```python
from build123d import *

# Parameters (mm, degrees)
SKETCH_1_W           = 88
SKETCH_1_H           = 58
EXTRUDE_1_DEPTH      = 18.8
SKETCH_2_W           = 7
SKETCH_2_H           = 7
CUT_EXTRUDE_1_DEPTH  = 15
SKETCH_3_R           = 1.55
CUT_EXTRUDE_2_DEPTH  = 3
SKETCH_4_W           = 72
SKETCH_4_H           = 42
CUT_EXTRUDE_6_DEPTH  = 16
SKETCH_6_W           = 16
SKETCH_6_H           = 8
CUT_EXTRUDE_7_DEPTH  = 8
CUT_EXTRUDE_11_REACH = 109.058
SKETCH_7_W           = 13
SKETCH_7_H           = 7
SKETCH_7_W_2         = 7
SKETCH_7_H_2         = 12
SKETCH_7_W_3         = 12
CUT_EXTRUDE_13_REACH = 109.058
SKETCH_10_W          = 8
SKETCH_10_H          = 16
CUT_EXTRUDE_14_REACH = 108.457
SKETCH_3_2_R         = 1.55
SKETCH_14_W          = 0.5
SKETCH_14_H          = 1.75
SKETCH_14_H_2        = 0.5
SKETCH_14_W_2        = 1.75
SKETCH_14_W_3        = 4
EXTRUDE_3_DEPTH      = 1
SKETCH_16_W          = 4
SKETCH_16_H          = 0.5
SKETCH_16_W_2        = 0.5
SKETCH_16_H_2        = 4
EXTRUDE_5_DEPTH      = 1
SKETCH_18_W          = 4
SKETCH_18_H          = 0.5
SKETCH_18_W_2        = 0.5
SKETCH_18_H_2        = 4
EXTRUDE_6_DEPTH      = 1


with BuildPart() as part:
    # Sketch 1 → Extrude 1 (new body)
    with BuildSketch(Plane.XY):
        with Locations((44, 29)):
            Rectangle(SKETCH_1_W, SKETCH_1_H)
    extrude(amount=EXTRUDE_1_DEPTH)

    # Sketch 2 → Cut-Extrude 1 (cut)
    with BuildSketch(Plane.XY.offset(18.8)):
        with Locations((3.5, 54.5)):
            Rectangle(SKETCH_2_W, SKETCH_2_H)
        with Locations((3.5, 3.5)):
            Rectangle(SKETCH_2_W, SKETCH_2_H)
        with Locations((84.5, 3.5)):
            Rectangle(SKETCH_2_W, SKETCH_2_H)
        with Locations((84.5, 54.5)):
            Rectangle(SKETCH_2_W, SKETCH_2_H)
    extrude(amount=-CUT_EXTRUDE_1_DEPTH, mode=Mode.SUBTRACT)

    # Sketch 3 → Cut-Extrude 2 (cut)
    with BuildSketch(Plane.XY.offset(3.8)):
        with Locations((4, 54)):
            Circle(SKETCH_3_R)
        with Locations(Location((4, 4, 0), (0, 0, 180))):
            Circle(SKETCH_3_R)
        with Locations((84, 4)):
            Circle(SKETCH_3_R)
        with Locations(Location((84, 54, 0), (0, 0, 180))):
            Circle(SKETCH_3_R)
    extrude(amount=-CUT_EXTRUDE_2_DEPTH, mode=Mode.SUBTRACT)

    # Sketch 4 → Cut-Extrude 6 (cut)
    with BuildSketch(Plane(origin=(0, 0, 0), x_dir=(-1, 0, 0), z_dir=(0, 0, -1))):
        with Locations((-44, 29)):
            Rectangle(SKETCH_4_W, SKETCH_4_H)
    extrude(amount=-CUT_EXTRUDE_6_DEPTH, mode=Mode.SUBTRACT)

    # Sketch 6 → Cut-Extrude 7 (cut)
    with BuildSketch(Plane.XZ):
        with Locations((24, 4)):
            Rectangle(SKETCH_6_W, SKETCH_6_H)
    extrude(amount=-CUT_EXTRUDE_7_DEPTH, mode=Mode.SUBTRACT)

    # Sketch 7 → Cut-Extrude 11 (cut, up to next)
    with BuildSketch(Plane.XY.offset(18.8), mode=Mode.PRIVATE) as cut_extrude_11_sk1:
        with Locations((40.5, 41.5)):
            Rectangle(SKETCH_7_W, SKETCH_7_H)
    cut_extrude_11_tool1 = extrude(cut_extrude_11_sk1.sketch, amount=-CUT_EXTRUDE_11_REACH, mode=Mode.PRIVATE) & part.part
    # Sketch 7 → Cut-Extrude 11 (cut, up to next)
    with BuildSketch(Plane.XY.offset(18.8), mode=Mode.PRIVATE) as cut_extrude_11_sk2:
        with Locations((73.5, 34)):
            Rectangle(SKETCH_7_W_2, SKETCH_7_H_2)
    cut_extrude_11_tool2 = extrude(cut_extrude_11_sk2.sketch, amount=-CUT_EXTRUDE_11_REACH, mode=Mode.PRIVATE) & part.part
    # Sketch 7 → Cut-Extrude 11 (cut, up to next)
    with BuildSketch(Plane.XY.offset(18.8), mode=Mode.PRIVATE) as cut_extrude_11_sk3:
        with Locations((24, 14.5)):
            Rectangle(SKETCH_7_W_3, SKETCH_7_H)
    cut_extrude_11_tool3 = extrude(cut_extrude_11_sk3.sketch, amount=-CUT_EXTRUDE_11_REACH, mode=Mode.PRIVATE) & part.part
    add(cut_extrude_11_tool1.solids().sort_by_distance((40.5, 41.5, 18.8))[0], mode=Mode.SUBTRACT)
    add(cut_extrude_11_tool2.solids().sort_by_distance((73.5, 34, 18.8))[0], mode=Mode.SUBTRACT)
    add(cut_extrude_11_tool3.solids().sort_by_distance((24, 14.5, 18.8))[0], mode=Mode.SUBTRACT)

    # Sketch 10 → Cut-Extrude 13 (cut, up to next)
    with BuildSketch(Plane(origin=(88, 0, 0), x_dir=(0, 0, -1), z_dir=(1, 0, 0)), mode=Mode.PRIVATE) as cut_extrude_13_sk1:
        with Locations((-4, 34)):
            Rectangle(SKETCH_10_W, SKETCH_10_H)
    cut_extrude_13_tool1 = extrude(cut_extrude_13_sk1.sketch, amount=-CUT_EXTRUDE_13_REACH, mode=Mode.PRIVATE) & part.part
    add(cut_extrude_13_tool1.solids().sort_by_distance((88, 34, 4))[0], mode=Mode.SUBTRACT)

    # Sketch 3_2 → Cut-Extrude 14 (cut, up to next)
    with BuildSketch(Plane.XY.offset(3.8), mode=Mode.PRIVATE) as cut_extrude_14_sk1:
        with Locations((4, 54)):
            Circle(SKETCH_3_2_R)
    cut_extrude_14_tool1 = extrude(cut_extrude_14_sk1.sketch, amount=-CUT_EXTRUDE_14_REACH, mode=Mode.PRIVATE) & part.part
    # Sketch 3_2 → Cut-Extrude 14 (cut, up to next)
    with BuildSketch(Plane.XY.offset(3.8), mode=Mode.PRIVATE) as cut_extrude_14_sk2:
        with Locations((4, 4)):
            Circle(SKETCH_3_2_R)
    cut_extrude_14_tool2 = extrude(cut_extrude_14_sk2.sketch, amount=-CUT_EXTRUDE_14_REACH, mode=Mode.PRIVATE) & part.part
    # Sketch 3_2 → Cut-Extrude 14 (cut, up to next)
    with BuildSketch(Plane.XY.offset(3.8), mode=Mode.PRIVATE) as cut_extrude_14_sk3:
        with Locations((84, 4)):
            Circle(SKETCH_3_2_R)
    cut_extrude_14_tool3 = extrude(cut_extrude_14_sk3.sketch, amount=-CUT_EXTRUDE_14_REACH, mode=Mode.PRIVATE) & part.part
    # Sketch 3_2 → Cut-Extrude 14 (cut, up to next)
    with BuildSketch(Plane.XY.offset(3.8), mode=Mode.PRIVATE) as cut_extrude_14_sk4:
        with Locations((84, 54)):
            Circle(SKETCH_3_2_R)
    cut_extrude_14_tool4 = extrude(cut_extrude_14_sk4.sketch, amount=-CUT_EXTRUDE_14_REACH, mode=Mode.PRIVATE) & part.part
    add(cut_extrude_14_tool1.solids().sort_by_distance((4, 54, 3.8))[0], mode=Mode.SUBTRACT)
    add(cut_extrude_14_tool2.solids().sort_by_distance((4, 4, 3.8))[0], mode=Mode.SUBTRACT)
    add(cut_extrude_14_tool3.solids().sort_by_distance((84, 4, 3.8))[0], mode=Mode.SUBTRACT)
    add(cut_extrude_14_tool4.solids().sort_by_distance((84, 54, 3.8))[0], mode=Mode.SUBTRACT)

    # Sketch 14 → Extrude 3 (add)
    with BuildSketch(Plane.XY.offset(18.8)):
        with Locations((20, 8.125)):
            Rectangle(SKETCH_14_W, SKETCH_14_H)
        with Locations((20, 7)):
            Rectangle(SKETCH_14_W, SKETCH_14_H_2)
        with Locations((18.875, 7)):
            Rectangle(SKETCH_14_W_2, SKETCH_14_H_2)
        with Locations((21.125, 7)):
            Rectangle(SKETCH_14_W_2, SKETCH_14_H_2)
        with Locations((20, 5.875)):
            Rectangle(SKETCH_14_W, SKETCH_14_H)
        with Locations((28, 7)):
            Rectangle(SKETCH_14_W_3, SKETCH_14_H_2)
    extrude(amount=EXTRUDE_3_DEPTH)

    # Sketch 16 → Extrude 5 (add)
    with BuildSketch(Plane.XY.offset(18.8)):
        with Locations((65.982583839, 37.800395287)):
            Rectangle(SKETCH_16_W, SKETCH_16_H)
        with Locations((65.982583839, 37.800395287)):
            Rectangle(SKETCH_16_W_2, SKETCH_16_H_2)
        with Locations((65.982583839, 30.12335271)):
            Rectangle(SKETCH_16_W, SKETCH_16_H)
    extrude(amount=EXTRUDE_5_DEPTH)

    # Sketch 18 → Extrude 6 (add)
    with BuildSketch(Plane.XY.offset(18.8)):
        with Locations((31.020756215, 41.775617215)):
            Rectangle(SKETCH_18_W, SKETCH_18_H)
        with Locations((31.020756215, 41.775617215)):
            Rectangle(SKETCH_18_W_2, SKETCH_18_H_2)
        with Locations((49.451487349, 41.714982736)):
            Rectangle(SKETCH_18_W, SKETCH_18_H)
    extrude(amount=EXTRUDE_6_DEPTH)


solid = part.part
```
Build history of the part. All positions in model axes, mm. A direction names the side the tool comes from. Round coordinates to 2 decimals unless told otherwise and drop trailing zeros. Write each loop counter-clockwise with the first axis right and the second up, starting at its lowest first coordinate (ties: lowest second). Pieces come first, ordered by that corner, then holes. Notation, with made-up numbers: (50.5, 29.25) - (55.5, 29.25) arc R23 ccw to (55.5, 50.25) - close; hole circle Ø3 at (-28, 28). An arc over 180 degrees is marked (long way). Write each question's results on one line, items separated by ' | '. Start each with the question number.
Item 1: Wall check: L1, parallel to Y at x = 4, z = 2; L2, parallel to Y at x = 84, z = 3.2; L3, parallel to Y at x = 53, z = 13.25. Give the ranges that are in metal, low to high. Write a range as [from, to].
Item 2: Saw through at C-C (z = 7). Write the cut outline in (x, y).
Item 3: Saw through at B-B (y = 54). Write the cut outline in (x, z), and give its area (3 significant figures).
Item 4: Saw through at A-A (x = 84). Write the cut outline in (y, z), and give its area (3 significant figures).
Item 5: Which spindle directions (+Z, -Z, +X, -X, +Y, -Y) get a long thin tool onto all of the face, cutting with end or side? Do faces 1 (the face through (84, 42, 4)), 2 (the face through (24, 4, 8)), 3 (the face through (45, 50, 8)), 4 (the face through (24, 18, 17)). Say none if no direction does.
Item 6: Drop flat-ended pins along their axis: P1, Ø6, axis at x = 78, y = 14, coming from the +Z side; P2, Ø5.5, axis at x = 86, z = 15, coming from the -Y side; P3, Ø2, axis at y = 56, z = 13, coming from the +X side; P4, Ø3, axis at x = 84, y = 4, coming from the +Z side. Give the stop position or say it passes through.
Item 7: Saw through at D-D (x = 27). Write the cut outline in (y, z), and give its area (3 significant figures).
Item 8: Mould opens along X. For faces 5 (the face through (0, 29, 9)), 6 (the face through (3.798, 55.537, 1.927)), 7 (the face through (18, 14, 17)), 8 (the face through (66, 38, 19.8)) say: pulls with the +X half, pulls with the -X half, needs draft (parallel to the pull), parting line crosses it, or undercut.
Results are:
1) L1: y = [0, 2.45], [5.55, 52.45], [55.55, 58] | L2: y = [0, 2.45], [5.55, 26], [42, 52.45], [55.55, 58] | L3: y = [0, 8], [50, 58]
2) outline: (0, 7) - (7, 7) - (7, 0) - (16, 0) - (16, 8) - (8, 8) - (8, 50) - (80, 50) - (80, 42) - (88, 42) - (88, 51) - (81, 51) - (81, 58) - (7, 58) - (7, 51) - (0, 51) - close; (32, 0) - (81, 0) - (81, 7) - (88, 7) - (88, 26) - (80, 26) - (80, 8) - (32, 8) - close
3) outline: (0, 0) - (2.45, 0) - (2.45, 3.8) - (0, 3.8) - close; (5.55, 0) - (82.45, 0) - (82.45, 3.8) - (81, 3.8) - (81, 18.8) - (7, 18.8) - (7, 3.8) - (5.55, 3.8) - close; (85.55, 0) - (88, 0) - (88, 3.8) - (85.55, 3.8) - close | area: 1,420 mm²
4) outline: (0, 0) - (2.45, 0) - (2.45, 3.8) - (0, 3.8) - close; (5.55, 0) - (26, 0) - (26, 8) - (42, 8) - (42, 0) - (52.45, 0) - (52.45, 3.8) - (51, 3.8) - (51, 18.8) - (7, 18.8) - (7, 3.8) - (5.55, 3.8) - close; (55.55, 0) - (58, 0) - (58, 3.8) - (55.55, 3.8) - close | area: 729 mm²
5) face 1: -Z, +X | face 2: -Z, -Y | face 3: -Z | face 4: +Z, -Z
6) P1: stops at z = 18.8 | P2: stops at y = 7 | P3: stops at x = 81 | P4: passes through
7) outline: (0, 8) - (8, 8) - (8, 16) - (11, 16) - (11, 18.8) - (7.25, 18.8) - (7.25, 19.8) - (6.75, 19.8) - (6.75, 18.8) - (0, 18.8) - close; (18, 16) - (50, 16) - (50, 0) - (58, 0) - (58, 18.8) - (18, 18.8) - close | area: 335 mm²
8) face 5: pulls with the -X half | face 6: undercut | face 7: undercut | face 8: needs draft
